Autodesk Inventor part; units mm, degrees
ref_plane "РабПлоскость1" through (0, 0, 0) normal (1, 0, 0) x (0, 0, -1)
ref_plane "YZ Plane" through (0, 0, 0) normal (1, 0, 0) x (0, 1, 0)
ref_plane "XZ Plane" through (0, 0, 0) normal (0, 1, 0) x (-1, 0, 0)
sketch "Эскиз1" plane through (0, 0, 0) normal (1, 0, 0) x (0, 1, 0)
  circle A0 centre (0, 0) radius 14
  dimension "d0" = 28
extrude "Выдавливание1" add sketch "Эскиз1" along normal mid plane 60
sketch "Эскиз2" plane through (30, 0, 0) normal (1, 0, 0) x (0, 0, -1)
  point P0 (0, 0)
  point P1 (0, 0)
hole "Отверстие1" at (30, 0, 0) direction (-1, 0, 0) diameter 3 depth 60
fillet "Сопряжение1" radius 0.2 2 edges at (30, 0, 1.5) (-30, 0, 1.5)
ref_plane "РабПлоскость1" through (0, 0, 0) normal (1, 0, 0) x (0, 0, -1)
sketch "Эскиз3" plane through (0, 0, 0) normal (1, 0, 0) x (0, 0, -1)
  circle A0 centre (0, 0) radius 12.5
  circle A1 centre (0, 0) radius 14
  dimension "d11" = 25
extrude "Выдавливание2" cut sketch "Эскиз3" along normal mid plane 10
properties part number "Вал конвейера"
The model under review builds one solid part; all positions refer to its coordinate system, in mm. A direction names the side the tool comes from. Round coordinates to 2 decimals unless told otherwise and drop trailing zeros. Write each loop counter-clockwise with the first axis right and the second up, starting at its lowest first coordinate (ties: lowest second). Pieces come first, ordered by that corner, then holes. Notation, with made-up numbers: (60, 8) - (118, 8) arc R15 cw to (118, 27) - close; hole circle Ø1 at (80, -26.75). An arc over 180 degrees is marked (long way). Use one line per item in the form item = value.
Q1. Draft analysis for pull direction X (two halves, no side actions). For faces 3 (the cylindrical face through (0.07, 3.755, -11.923)), 4 (the flat face through (30, 0, -3)), 5 (the flat face through (-30, 0, -3)), state which applies: +X half, -X half, draft (parallel to the pull), parting line (faces both ways), or undercut.
Answer key:
face_3 = undercut
face_4 = +X half
face_5 = -X half
Q2. Insertion check: pin 1 Ø12 at (x, z) = (-22.5, 10) entering from -Y; pin 2 Ø3 at (x, y) = (-1.5, -8) entering from -Z; pin 3 Ø1.5 at (x, z) = (-9, -10.5) entering from -Y. Each pin has a flat end and moves straight along its axis. Give the tip position at first contact, or say it passes through.
Answer key:
pin_1 = -13.42
pin_2 = -10.68
pin_3 = -10.05
Q3. Consider section D-D (y = 8.5). State the section outline as (x, z) points.
Answer key:
outline = (-30, -11.12) - (-5, -11.12) - (-5, -9.17) - (5, -9.17) - (5, -11.12) - (30, -11.12) - (30, 11.12) - (5, 11.12) - (5, 9.17) - (-5, 9.17) - (-5, 11.12) - (-30, 11.12) - close
Q4. For line 1 (Y direction, x = -4, z = 0); line 2 (Y direction, x = -7.5, z = 0), list the stretches that pass through material, from the lowest coordinate up. Write a range as [from, to].
Answer key:
line_1 = [-12.5, -1.5], [1.5, 12.5]
line_2 = [-14, -1.5], [1.5, 14]
Q5. Consider section A-A (y = 0). State the section outline as (x, z) points.
Answer key:
outline = (-30, -14) - (-5, -14) - (-5, -12.5) - (5, -12.5) - (5, -14) - (30, -14) - (30, -1.7) arc R0.2 ccw to (29.8, -1.5) - (-29.8, -1.5) arc R0.2 ccw to (-30, -1.7) - close; (-30, 1.7) arc R0.2 ccw to (-29.8, 1.5) - (29.8, 1.5) arc R0.2 ccw to (30, 1.7) - (30, 14) - (5, 14) - (5, 12.5) - (-5, 12.5) - (-5, 14) - (-30, 14) - close
Q6. Consider section C-C (x = 22). State the section outline as (y, z) points.
Answer key:
outline = circle Ø28 at (0, 0); hole circle Ø3 at (0, 0)
Q7. Tool access review of faces 1 (the cylindrical face through (17.325, 12.932, 5.362)), 2 (the flat face through (-5, 11.5, 5.3)): name each direction out of +Z, -Z, +X, -X, +Y, -Y from which nothing blocks a thin tool from reaching the whole face with its end or side.
Answer key:
face_1 = +X, -X
face_2 = none
